Geometry check sheet. Reference: the model listing, model coordinates, mm. A direction names the side the tool comes from. Coordinates: 2 decimals unless noted, no trailing zeros. Put each result on its own line as item: value. Start each with the question number.
1) Mould release check, pull along Y, two halves, no side actions. Record for faces 3 (the conical face through (214.289, -243.142, 1.875)), 4 (the flat face through (108.9, -250.705, 2.7)), 5 (the flat face through (65, -244, 3)), 6 (the conical face through (286.789, -243.142, 1.875)): released by +Y, released by -Y, zero draft, split by the parting line, or undercut.
2) Set-up check for faces 1 (the flat face through (310, -244, 3)), 2 (the cylindrical face through (106.545, -243.607, 4.138)): record each of +Z, -Z, +X, -X, +Y, -Y from which the full face is reachable in a straight line by a thin tool's end or side.
3) Cross-section at A-A on z = 5.5. Count the separate pieces of the cut face and the enclosed holes in it, plus the area to 3 significant figures.
4) Gauge pin test, flat ends, axial feed: pin 1 (2 mm diameter, centred on x = 285, y = -243.7, fed in from +Z); pin 2 (1.5 mm diameter, centred on y = -251.5, z = 4, fed in from -X); pin 3 (4 mm diameter, centred on x = 162.5, y = -243.7, fed in from -Z); pin 4 (2.5 mm diameter, centred on y = -252.5, z = 3.5, fed in from +X). Record the tip position at first contact, or that the pin passes through.
5) Scan lines: line 1 along X through (y, z) = (-243.25, 2.25); line 2 along Y through (x, z) = (285, 5.75); line 3 along Y through (x, z) = (90, 5.55). Record each from-to range of solid material in increasing order.
from build123d import *

# Parameters (mm, degrees)
SKETCH085_W     = 245
SKETCH085_H     = 14
SKETCH085_R     = 1.75
PAD043_DEPTH    = 7
CHAMFER010_SIZE = 2
SKETCH086_W     = 155.909408
SKETCH086_H     = 3
PAD044_DEPTH    = 7
SKETCH097_W     = 8
SKETCH097_H     = 22
POCKET043_DEPTH = 4
FILLET003_R     = 3.99


with BuildPart() as part:
    # Sketch085 → Pad043 (new body)
    with BuildSketch(Plane.XY):
        with Locations((187.5, -243.704939)):
            Rectangle(SKETCH085_W, SKETCH085_H)
        with Locations((162.5, -243.704939)):
            Circle(SKETCH085_R, mode=Mode.SUBTRACT)
        with Locations((90, -243.704939)):
            Circle(SKETCH085_R, mode=Mode.SUBTRACT)
        with Locations((212.5, -243.704939)):
            Circle(SKETCH085_R, mode=Mode.SUBTRACT)
        with Locations((285, -243.704939)):
            Circle(SKETCH085_R, mode=Mode.SUBTRACT)
    extrude(amount=PAD043_DEPTH)

    # Chamfer010
    chamfer010_edges = [part.edges().sort_by_distance(p)[0] for p in [
        (283.25, -243.704939, 0),
        (210.75, -243.704939, 0),
        (160.75, -243.704939, 0),
        (88.25, -243.704939, 0),
    ]]
    chamfer(chamfer010_edges, length=CHAMFER010_SIZE)

    # Sketch086 → Pad044 (join)
    with BuildSketch(Plane.XY):
        with Locations((232.026436, -252.13768)):
            Rectangle(SKETCH086_W, SKETCH086_H)
    extrude(amount=PAD044_DEPTH)

    # Sketch097 (on DatumPlane) → Pocket043 (cut)
    with BuildSketch(Plane.XY.offset(7)):
        with Locations((109.345456, -244.63761)):
            Rectangle(SKETCH097_W, SKETCH097_H)
    extrude(amount=-POCKET043_DEPTH, mode=Mode.SUBTRACT)

    # Fillet003
    fillet003_edges = [part.edges().sort_by_distance(p)[0] for p in [
        (113.345456, -243.704939, 3),
        (105.345456, -243.704939, 3),
    ]]
    fillet(fillet003_edges, radius=FILLET003_R)


solid = part.part
Answer key:
1. face 3: undercut
1. face 4: released by -Y
1. face 5: zero draft
1. face 6: undercut
2. face 1: +Z, -Z, +X, +Y, -Y
2. face 2: +Z, +Y, -Y
3. separate pieces: 2
3. enclosed holes: 4
3. area: 3,740 mm²
4. pin 1: passes through
4. pin 2: stops at x = 154.07
4. pin 3: stops at z = 1.75
4. pin 4: stops at x = 309.98
5. line 1: x = 65 to 88.31, 91.69 to 160.81, 164.19 to 210.81, 214.19 to 283.31, 286.69 to 310
5. line 2: y = -253.64 to -245.45, -241.95 to -236.7
5. line 3: y = -250.7 to -245.45, -241.95 to -236.7
